Autodesk Inventor part; units mm, degrees
ref_plane "YZ Plane" through (0, 0, 0) normal (1, 0, 0) x (0, 1, 0)
ref_plane "XZ Plane" through (0, 0, 0) normal (0, 1, 0) x (-1, 0, 0)
ref_plane "XY Plane" through (0, 0, 0) normal (0, 0, 1) x (1, 0, 0)
sketch "Sketch2" plane through (0, 0, 0) normal (0, 0, 1) x (1, 0, 0)
  circle A0 centre (0, 0) radius 7.5
  dimension "d0" = 15
extrude "Extrusion1" add sketch "Sketch2" along normal blind 2
sketch "Sketch3" plane through (0, 0, 2) normal (0, 0, 1) x (1, 0, 0)
  circle A0 centre (0, 0) radius 7.5
  circle A1 centre (0, 0) radius 5.5
  dimension "d3" = 11
extrude "Extrusion2" add sketch "Sketch3" along normal blind 15 contours A1
sketch "Sketch4" plane through (0, 0, 0) normal (0, 0, -1) x (-1, 0, 0)
  circle A0 centre (0, 0) radius 7.5
hole "Hole1" at (0, 0, 0) direction (0, 0, 1) diameter 4.305 end through all
ref_plane "Work Plane1" through (0, 0, 16) normal (0, 0, 1) x (1, 0, 0)
sketch "Sketch5" plane through (0, 0, 0) normal (0, 0, -1) x (-1, 0, 0)
  circle A0 centre (0, 0) radius 2.1525
  circle A1 centre (0, 0) radius 7.5
  line L0 (2.4357, 4.2187) -> (4.8714, 0)
  line L1 (4.8714, 0) -> (2.4357, -4.2188)
  line L2 (2.4357, -4.2188) -> (-2.4357, -4.2187)
  line L3 (-2.4357, -4.2187) -> (-4.8714, 0)
  line L4 (-4.8714, 0) -> (-2.4357, 4.2187)
  line L5 (-2.4357, 4.2187) -> (2.4357, 4.2187)
  dimension "d14" = 8.4375
extrude "Extrusion3" cut sketch "Sketch5" against normal up to surface (16 mm away) contours L0 L1 L2 L3 L4 L5
sketch "Sketch6" plane through (0, 0, 0) normal (0, 0, -1) x (-1, 0, 0)
  line L0 (2.4357, -4.2188) -> (-2.4357, -4.2187)
  line L1 (-2.4357, -4.2187) -> (-4.8714, 0)
  line L2 (-4.8714, 0) -> (-2.4357, 4.2187)
  line L3 (-2.4357, 4.2187) -> (2.4357, 4.2187)
  line L4 (2.4357, 4.2187) -> (4.8714, 0)
  line L5 (4.8714, 0) -> (2.4357, -4.2188)
  circle A0 centre (0, 0) radius 7.5
  circle A1 centre (0, 0) radius 4 construction
  dimension "d17" = 8
sketch "Sketch7" plane through (0, 0, 0) normal (1, 0, 0) x (0, 1, 0)
  line L0 (-7.5, 0) -> (-7.5, 2)
  line L1 (-7.5, 2) -> (-5.5, 2)
  line L2 (-5.5, 2) -> (-5.5, 17)
  line L3 (-5.5, 17) -> (-2.1525, 17)
  line L4 (-2.1525, 17) -> (-2.1525, 16)
  line L5 (-2.1525, 16) -> (-4.2188, 16)
  line L6 (-4.2188, 16) -> (-4.2188, 0)
  line L7 (-4.2188, 0) -> (-7.5, 0)
  line L8 (7.5, 2) -> (7.5, 0)
  line L9 (7.5, 0) -> (4.2187, 0)
  line L10 (4.2187, 0) -> (4.2187, 16)
  line L11 (4.2187, 16) -> (2.1525, 16)
  line L12 (2.1525, 16) -> (2.1525, 17)
  line L13 (2.1525, 17) -> (5.5, 17)
  line L14 (5.5, 17) -> (5.5, 2)
  line L15 (5.5, 2) -> (7.5, 2)
  line L16 (2.1525, 16) -> (4.2187, 13.9338)
  line L17 (0, -3.4) -> (0, 20.4)
  point P0 (0, 0)
  dimension "d18" = 45
revolve "Revolution1" add sketch "Sketch7" angle 360 about axis through (0, 0, -10) along (0, 0, 1) contours L16 L11 L10
properties part number "z-keeper"
Source: CAD feature listing. Evaluate the final solid. Frame: model axes, mm. A direction names the side the tool comes from. Give positions to 0.01 mm unless a question says otherwise; leave off trailing zeros. Order: outer loops, then holes, each group sorted by start corner. A loop starts at its lowest first (then second) coordinate and runs counter-clockwise, first axis right, second up.
(1) Pull-direction query (Y, two-part tool) for faces 3 (the face through (-2.134, -0.28, 16.507)), 4 (the face through (-1.19, 5.37, 9.4)), 5 (the face through (3.2, -3.2, 0)), 6 (the face through (-3.67, -2.08, 7.89)); classes: +Y half, -Y half, draft (parallel to the pull), parting line (faces both ways), or undercut.
(2) Section query B-B (x = 5.25). Return the cut outline in (y, z).
(3) Contact query for flat-ended pins moving along their axis: P1, Ø8, axis at x = -4, z = 8, coming from the +Y side; P2, Ø1, axis at y = 5, z = 5, coming from the -X side; P3, Ø1, axis at x = 2, y = 3, coming from the -Z side. Output: stop coordinate, or through.
(4) Access query for faces 1 (the face through (0.685, 2.176, 15.871)), 2 (the face through (-4, 4, 2)). Directions: +Z, -Z, +X, -X, +Y, -Y. A direction counts if a zero-diameter tool reaches every point of the face in a straight line with its end or side. Return the directions, or none.
(5) Section query A-A (z = 5.25). Return the cut outline in (x, y), plus the area to 3 significant figures.
(6) Material intervals for line 1 along Y through (x, z) = (0, 16.85); line 2 along Z through (x, y) = (-1, -5.5); line 3 along Y through (x, z) = (2, 11.25), sorted ascending.
Outcome:
1. face 3: undercut
1. face 4: parting line
1. face 5: draft
1. face 6: undercut
2. outline: (-5.36, 0) - (5.36, 0) - (5.36, 2) - (1.64, 2) - (1.64, 17) - (-1.64, 17) - (-1.64, 2) - (-5.36, 2) - close
3. P1: stops at y = 5.5
3. P2: stops at x = -3.16
3. P3: stops at z = 14.05
4. face 1: -Z
4. face 2: +Z
5. outline: circle Ø11 at (0, 0); hole (-4.87, 0) - (-2.44, -4.22) - (2.44, -4.22) - (4.87, 0) - (2.44, 4.22) - (-2.44, 4.22) - close
5. area: 33.4 mm2
6. line 1: y = -5.5 to -2.15, 2.15 to 5.5
6. line 2: z = 0 to 2
6. line 3: y = -5.12 to -4.22, 4.22 to 5.12
